Work out the finished part from the listing and answer in its coordinate system (mm). A direction names the side the tool comes from. Round coordinates to 2 decimals unless told otherwise and drop trailing zeros. Write each loop counter-clockwise with the first axis right and the second up, starting at its lowest first coordinate (ties: lowest second). Pieces come first, ordered by that corner, then holes.
from build123d import *

# Parameters (mm, degrees)
BOSS_EXTRU_1_DEPTH         = 20
ESQUISSE2_R                = 4
ENL_V_MAT_EXTRU_1_DEPTH    = 811.740402348
R_P_TITION_LIN_AIRE1_COUNT = 8
R_P_TITION_LIN_AIRE1_PITCH = 100
ESQUISSE3_R                = 7.5
ENL_V_MAT_EXTRU_2_DEPTH    = 10


with BuildPart() as part:
    # Esquisse1 → Boss.-Extru.1 (new body)
    with BuildSketch(Plane.XY):
        Polygon((0, 130), (0, 120), (790, 120), (790, 10), (0, 10), (0, 0), (800, 0), (800, 130), align=None)
    extrude(amount=BOSS_EXTRU_1_DEPTH)

    # Esquisse2 → Enlèv. mat.-Extru.1 (cut, through all)
    with BuildSketch(Plane(origin=(0, 130, 0), x_dir=(1, 0, 0), z_dir=(0, 1, 0))):
        with Locations(Location((20, -10, 0), (0, 0, 270))):
            Circle(ESQUISSE2_R)
    enl_v_mat_extru_1 = extrude(amount=-ENL_V_MAT_EXTRU_1_DEPTH, mode=Mode.SUBTRACT)

    # Répétition linéaire1: Enlèv. mat.-Extru.1 ×8
    with Locations(*[(i * R_P_TITION_LIN_AIRE1_PITCH, 0, 0) for i in range(1, R_P_TITION_LIN_AIRE1_COUNT)]):
        add(enl_v_mat_extru_1, mode=Mode.SUBTRACT)

    # Esquisse3 → Enlèv. mat.-Extru.2 (cut)
    with BuildSketch(Plane(origin=(0, 130, 0), x_dir=(1, 0, 0), z_dir=(0, 1, 0))):
        with Locations(Location((370, -10, 0), (0, 0, 270))):
            Circle(ESQUISSE3_R)
    extrude(amount=-ENL_V_MAT_EXTRU_2_DEPTH, mode=Mode.SUBTRACT)


solid = part.part
Q1. Given pin 1 (2 mm diameter, centred on y = 80.5, z = 16.5, fed in from -X), flat-ended and moving along its own axis, determine where the tip first touches the part or whether it passes through.
Q2. A tool of negligible diameter and unlimited length cuts with its end or side. For faces 5 (the face through (800, 64, 10)), 6 (the face through (790, 66, 10)), from which of +Z, -Z, +X, -X, +Y, -Y can it reach the whole face along a straight path? Write none if from no direction.
Q3. Find section A-A (x = 261.5). Determine the outline of the cut face in (y, z).
Q4. Find section B-B (z = 10). Count the separate pieces of the cut face and the enclosed holes in it, plus the area to 3 significant figures.
Q5. Find the intervals of material crossed by L1, parallel to Y at x = 38, z = 7.75; L2, parallel to Z at x = 620, y = 8; L3, parallel to X at y = 55.5, z = 6.5, in increasing order.
Q6. Find section C-C (y = 87). Determine the outline of the cut face in (x, z), plus the area to 3 significant figures.
Q7. The mould has two halves that part along Z. Classify faces 1 (the face through (398, 123, 20)), 2 (the face through (398, 123, 0)), 3 (the face through (362.68, 125.07, 8.37)), 4 (the face through (389, 120, 10)): +Z half, -Z half, draft (parallel to the pull), parting line (faces both ways), or undercut.
Report:
1. pin 1: stops at x = 790
2. face 5: +Z, -Z, +X, +Y, -Y
2. face 6: +Z, -Z, -X
3. outline: (0, 0) - (10, 0) - (10, 20) - (0, 20) - close; (120, 0) - (130, 0) - (130, 20) - (120, 20) - close
4. separate pieces: 18
4. enclosed holes: 0
4. area: 15,700 mm2
5. L1: y = 0 to 10, 120 to 130
5. L2: z = 0 to 6, 14 to 20
5. L3: x = 790 to 800
6. outline: (790, 0) - (800, 0) - (800, 20) - (790, 20) - close
6. area: 200 mm2
7. face 1: +Z half
7. face 2: -Z half
7. face 3: undercut
7. face 4: draft
